Part model, mm, in its own coordinate system. Face numbers are marked on the shaded views. Give positions to 0.01 mm unless a question says otherwise; leave off trailing zeros. Order: outer loops, then holes, each group sorted by start corner. A loop starts at its lowest first (then second) coordinate and runs counter-clockwise, first axis right, second up. Notation, with made-up numbers: (67.5, -19) - (84.5, -19) arc R7 ccw to (84.5, -14) - close; hole circle Ø9 at (78, 73.25). An arc over 180 degrees is marked (long way). Use a Markdown table: item, result. Add a question column.
from build123d import *

# Parameters (mm, degrees)
SALIENTE_EXTRUIR2_DEPTH                     = 5
REFRENTADO_PARA_TORNILLO_CON_CABEZA_2_COUNT = 2
REFRENTADO_PARA_TORNILLO_CON_CABEZA_2_PITCH = 180
REFRENTADO_PARA_TORNILLO_CON_CABEZA_3_COUNT = 2
REFRENTADO_PARA_TORNILLO_CON_CABEZA_3_PITCH = 240.831891576
REFRENTADO_PARA_TORNILLO_CON_CABEZA_4_COUNT = 2
REFRENTADO_PARA_TORNILLO_CON_CABEZA_4_PITCH = 160
CORTAR_EXTRUIR1_DEPTH                       = 2
CROQUIS8_W                                  = 10
CROQUIS8_H                                  = 10
SALIENTE_EXTRUIR7_DEPTH                     = 5
TALADRO_DE_MARGEN_PARA_M31_D                = 3.2
TALADRO_DE_MARGEN_PARA_M31_DEPTH            = 5
TALADRO_DE_MARGEN_PARA_M31_TIP              = 0.96137699


with BuildPart() as part:
    # Croquis1 → Saliente-Extruir2 (new body)
    with BuildSketch(Plane(origin=(0, 0, 0), x_dir=(1, 0, 0), z_dir=(0, 1, 0))):
        with BuildLine():
            Line((-79.5, -94.5), (79.5, -94.5))
            ThreePointArc((79.5, -94.5), (83.035533906, -93.035533906), (84.5, -89.5))
            Line((84.5, -89.5), (84.5, 89.5))
            ThreePointArc((84.5, 89.5), (83.035533906, 93.035533906), (79.5, 94.5))
            Line((79.5, 94.5), (-79.5, 94.5))
            ThreePointArc((-79.5, 94.5), (-83.035533906, 93.035533906), (-84.5, 89.5))
            Line((-84.5, 89.5), (-84.5, -89.5))
            ThreePointArc((-84.5, -89.5), (-83.035533906, -93.035533906), (-79.5, -94.5))
        make_face()
    extrude(amount=SALIENTE_EXTRUIR2_DEPTH)

    # Croquis5 → Refrentado para tornillo con cabeza troncocónica de M31 (revolve, cut)
    with BuildSketch(Plane(origin=(80, 5, -90), x_dir=(0, 0, 1), z_dir=(1, 0, 0))):
        Polygon((0, 0), (0, 5), (1.6, 5), (1.6, 2.4), (3.5, 2.4), (3.5, -2), (1.5, 0), align=None)
    refrentado_para_tornillo_con_cabeza_tron = revolve(axis=Axis((80, 11.35, -90), (0, -1, 0)), mode=Mode.SUBTRACT)

    # Refrentado para tornillo con cabeza  2: Refrentado para tornillo con cabeza troncocónica de M31 ×2
    with Locations(*[(0, 0, i * REFRENTADO_PARA_TORNILLO_CON_CABEZA_2_PITCH) for i in range(1, REFRENTADO_PARA_TORNILLO_CON_CABEZA_2_COUNT)]):
        add(refrentado_para_tornillo_con_cabeza_tron, mode=Mode.SUBTRACT)

    # Refrentado para tornillo con cabeza  3: Refrentado para tornillo con cabeza troncocónica de M31 ×2
    with Locations(*[Vector(-0.664363839, 0, 0.747409319) * (i * REFRENTADO_PARA_TORNILLO_CON_CABEZA_3_PITCH) for i in range(1, REFRENTADO_PARA_TORNILLO_CON_CABEZA_3_COUNT)]):
        add(refrentado_para_tornillo_con_cabeza_tron, mode=Mode.SUBTRACT)

    # Refrentado para tornillo con cabeza  4: Refrentado para tornillo con cabeza troncocónica de M31 ×2
    with Locations(*[(-i * REFRENTADO_PARA_TORNILLO_CON_CABEZA_4_PITCH, 0, 0) for i in range(1, REFRENTADO_PARA_TORNILLO_CON_CABEZA_4_COUNT)]):
        add(refrentado_para_tornillo_con_cabeza_tron, mode=Mode.SUBTRACT)

    # Croquis6 → Cortar-Extruir1 (cut)
    with BuildSketch(Plane.XZ):
        Polygon((-81, 84), (-74, 91), (74, 91), (81, 84), (81, -84), (74, -91), (-74, -91), (-81, -84), align=None)
    extrude(amount=-CORTAR_EXTRUIR1_DEPTH, mode=Mode.SUBTRACT)

    # Croquis8 → Saliente-Extruir7 (add)
    with BuildSketch(Plane.XZ.offset(-2)):
        with Locations((-76, 79)):
            Rectangle(CROQUIS8_W, CROQUIS8_H)
        with Locations((76, 79)):
            Rectangle(CROQUIS8_W, CROQUIS8_H)
        with Locations((-76, -79)):
            Rectangle(CROQUIS8_W, CROQUIS8_H)
        with Locations((76, -79)):
            Rectangle(CROQUIS8_W, CROQUIS8_H)
    extrude(amount=SALIENTE_EXTRUIR7_DEPTH)

    # Taladro de margen para M31
    with Locations(Plane(origin=(0, -3, 0), x_dir=(-1, 0, 0), z_dir=(0, -1, 0))):
        with Locations((-76, 79), (76, 79), (76, -79), (-76, -79)):
            Hole(TALADRO_DE_MARGEN_PARA_M31_D / 2, depth=TALADRO_DE_MARGEN_PARA_M31_DEPTH)
            with Locations((0, 0, -(TALADRO_DE_MARGEN_PARA_M31_DEPTH + TALADRO_DE_MARGEN_PARA_M31_TIP / 2))):  # 118° drill point
                Cone(0, TALADRO_DE_MARGEN_PARA_M31_D / 2, TALADRO_DE_MARGEN_PARA_M31_TIP, mode=Mode.SUBTRACT)


solid = part.part
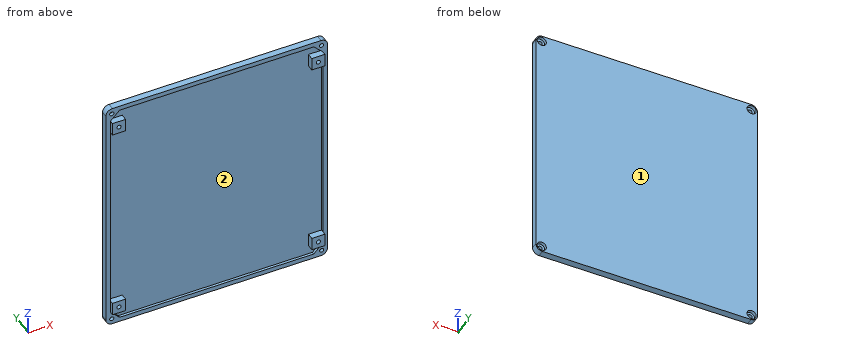
1. Cut at B-B (z = 18). Write the cut outline in (x, y), plus the area to 3 significant figures.
2. Drill centre lines: probe 1 along Z at (x, y) = (80, 3.3); probe 2 along X at (y, z) = (4.4, 90); probe 3 along Z at (x, y) = (-76, -0.55). Where is each one in solid material? Low to high. Write a range as [from, to].
3. Pin check, flat tips, straight feed: P1, Ø3.5, axis at x = 79.5, z = -91.5, coming from the +Y side; P2, Ø11, axis at x = -80, z = -90, coming from the -Y side; P3, Ø3, axis at x = 80, z = 90, coming from the +Y side; P4, Ø1.9, axis at x = 76, z = -79, coming from the -Y side. Stop position of each tip, or through.
4. Cut at A-A (x = 54.5). Write the cut outline in (y, z).
5. Mould opens along X. For the marked faces 1 and 2 say: released by +X, released by -X, zero draft, split by the parting line, or undercut.
Responses:
| question | item | result |
|---|---|---|
| 1 | outline | (-84.5, 0) - (-81, 0) - (-81, 2) - (81, 2) - (81, 0) - (84.5, 0) - (84.5, 5) - (-84.5, 5) - close |
| 1 | area | 521 mm² |
| 2 | probe 1 | z = [-94.47, -93.5], [-86.5, 86.5], [93.5, 94.47] |
| 2 | probe 2 | x = [-84.47, -83.5], [-76.5, 76.5], [83.5, 84.47] |
| 2 | probe 3 | z = [-84, -80.6], [-77.4, -74], [74, 77.4], [80.6, 84] |
| 3 | P1 | stops at y = 2.6 |
| 3 | P2 | stops at y = 0 |
| 3 | P3 | passes through |
| 3 | P4 | stops at y = 2.39 |
| 4 | outline | (0, -94.5) - (5, -94.5) - (5, 94.5) - (0, 94.5) - (0, 91) - (2, 91) - (2, -91) - (0, -91) - close |
| 5 | face 1 | zero draft |
| 5 | face 2 | undercut |
